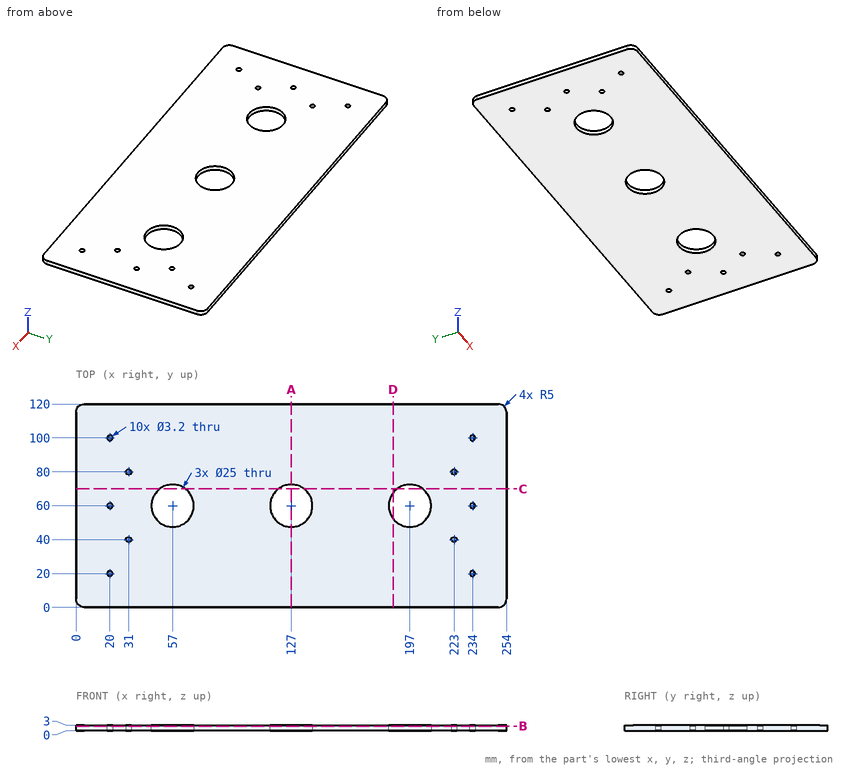
Print and shaded views of the part. All mm, measured from the part's lowest x, y and z. Coordinates: 2 decimals unless noted, no trailing zeros. Loops run counter-clockwise (first coordinate to the right, second up) from the corner with the lowest first, then second, coordinate; pieces in that order, holes last. Notation, with made-up numbers: (81, 12.5) -> (98, 12.5) arc R17 cw to (98, 27.5) -> close; hole circle Ø10 at (-31, 87). An arc over 180 degrees is marked (long way). Use a Markdown table: item, result. Add a question column.
Item 1: Flat gauge pin, fed straight in: P1, Ø2.5, axis at x = 20, y = 60, coming from the +Z side. Where does the tip first touch, or does it go through?
Item 2: Band-saw the part on D-D on x = 187. Write the cut outline in (y, z), plus the area to 3 significant figures.
Item 3: Probe probe 1 along Y at (x, z) = (20, 0.85); probe 2 along X at (y, z) = (40, 2.2); probe 3 along Y at (x, z) = (31, 1.65). List the from-to ranges inside material, lowest first.
Item 4: Band-saw the part on A-A on x = 127. Write the cut outline in (y, z), plus the area to 3 significant figures.
Item 5: Band-saw the part on B-B on z = 2.55. Give the number of separate pieces and of enclosed holes in the cut face, plus the area to 3 significant figures.
Item 6: Band-saw the part on C-C on y = 70. Write the cut outline in (x, z).
Geometry says:
| question | item | result |
|---|---|---|
| 1 | P1 | through |
| 2 | outline | (0, 0) -> (52.5, 0) -> (52.5, 3) -> (0, 3) -> close; (67.5, 0) -> (120, 0) -> (120, 3) -> (67.5, 3) -> close |
| 2 | area | 315 mm² |
| 3 | probe 1 | 0 to 18.4, 21.6 to 58.4, 61.6 to 98.4, 101.6 to 120 |
| 3 | probe 2 | 0 to 29.4, 32.6 to 221.4, 224.6 to 254 |
| 3 | probe 3 | 0 to 38.4, 41.6 to 78.4, 81.6 to 120 |
| 4 | outline | (0, 0) -> (47.5, 0) -> (47.5, 3) -> (0, 3) -> close; (72.5, 0) -> (120, 0) -> (120, 3) -> (72.5, 3) -> close |
| 4 | area | 285 mm² |
| 5 | separate pieces | 1 |
| 5 | enclosed holes | 13 |
| 5 | area | 28,900 mm² |
| 6 | outline | (0, 0) -> (49.5, 0) -> (49.5, 3) -> (0, 3) -> close; (64.5, 0) -> (119.5, 0) -> (119.5, 3) -> (64.5, 3) -> close; (134.5, 0) -> (189.5, 0) -> (189.5, 3) -> (134.5, 3) -> close; (204.5, 0) -> (254, 0) -> (254, 3) -> (204.5, 3) -> close |
